Can you work these out from the drawing? Everything is in mm from the part's minimum corner. A direction names the side the tool comes from. Give positions to 0.01 mm unless a question says otherwise; leave off trailing zeros. Order: outer loops, then holes, each group sorted by start corner. A loop starts at its lowest first (then second) coordinate and runs counter-clockwise, first axis right, second up. Notation, with made-up numbers: M 82.25,-29 L 104.25,-29 A32 cw 104.25,10 Z; hole C -8,-25 d3. An arc over 180 degrees is marked long. Use a Markdown table: item, result. Add a question column.
Item 1: I'm going to push flat-ended pins straight in: pin 1 Ø5 at (x, z) = (42.5, 6) entering from +Y; pin 2 Ø16 at (x, y) = (37.5, 35) entering from +Z; pin 3 Ø2 at (x, z) = (22.5, 18) entering from +Y; pin 4 Ø10 at (x, y) = (35.5, 45) entering from -Z. Where does each tip first touch, or does it pass through?
Item 2: Suppose I cut it at C-C on y = 42.5. Write out the boundary of the cut face in (x, z).
Item 3: If I drill on L1, parallel to Y at x = 12.5, z = 44.5; L2, parallel to Z at x = 10, y = 7.5; L3, parallel to Z at x = 46.5, y = 44, over which ranges is the centre line in solid material (lowest first)? Write a range as from..to.
Item 4: Suppose I cut it at D-D on z = 12. Write out the boundary of the cut face in (x, y).
Item 5: If we mould it in two halves opening along X, with no side actions, what happens to the marked faces 1, 2 and 3? For each: released by +X, released by -X, zero draft, split by the parting line, or undercut.
Item 6: Suppose I cut it at B-B on z = 19. Write out the boundary of the cut face in (x, y), plus the area to 3 significant figures.
Item 7: For the marked faces 4, 5, 6 and 7, which set-ups out of +Z, -Z, +X, -X, +Y, -Y let a thin tool reach every point of the face, with its end or its side?
Item 8: Suppose I cut it at A-A on y = 13. Write out the boundary of the cut face in (x, z), plus the area to 3 significant figures.
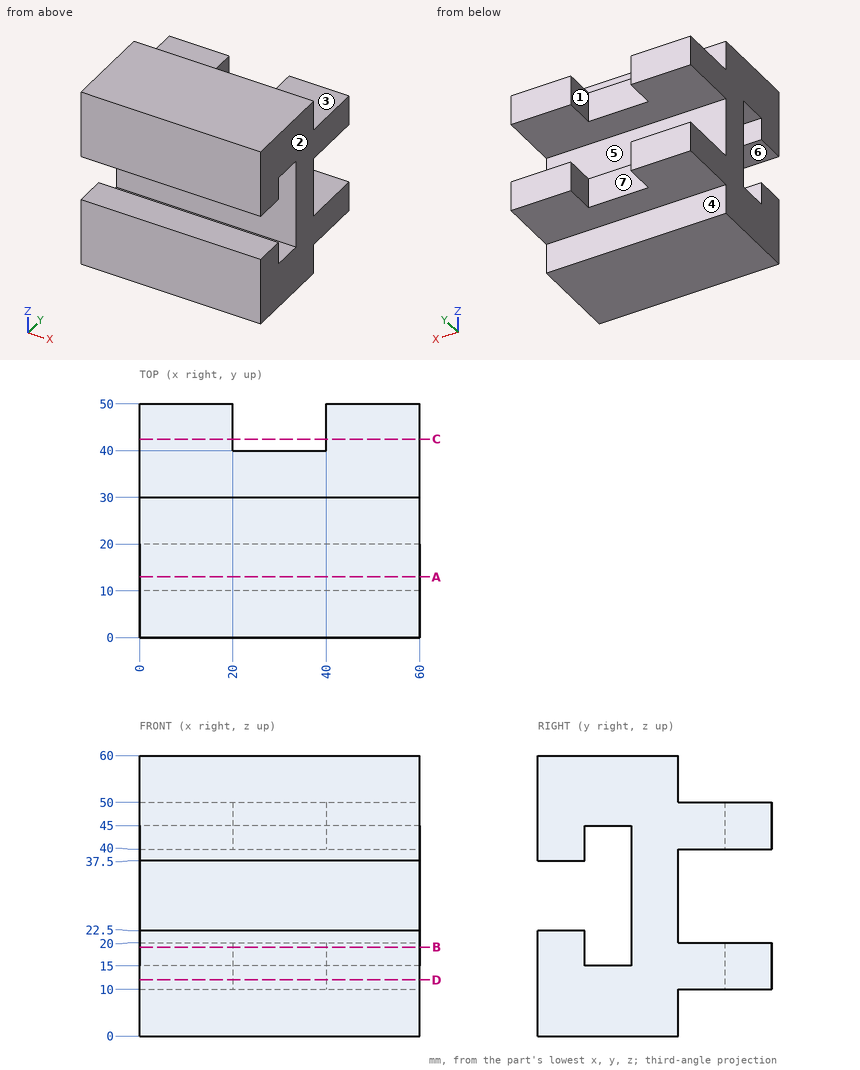
Findings below:
| question | item | result |
|---|---|---|
| 1 | pin 1 | stops at y = 30 |
| 1 | pin 2 | stops at z = 60 |
| 1 | pin 3 | stops at y = 40 |
| 1 | pin 4 | stops at z = 10 |
| 2 | outline | M 0,10 L 20,10 L 20,20 L 0,20 Z; M 0,40 L 20,40 L 20,50 L 0,50 Z; M 40,10 L 60,10 L 60,20 L 40,20 Z; M 40,40 L 60,40 L 60,50 L 40,50 Z |
| 3 | L1 | y = 0..10, 20..50 |
| 3 | L2 | z = 0..22.5, 37.5..60 |
| 3 | L3 | z = 10..20, 40..50 |
| 4 | outline | M 0,0 L 60,0 L 60,50 L 40,50 L 40,40 L 20,40 L 20,50 L 0,50 Z |
| 5 | face 1 | undercut |
| 5 | face 2 | released by +X |
| 5 | face 3 | zero draft |
| 6 | outline | M 0,0 L 60,0 L 60,10 L 0,10 Z; M 0,20 L 60,20 L 60,50 L 40,50 L 40,40 L 20,40 L 20,50 L 0,50 Z |
| 6 | area | 2,200 mm^2 |
| 7 | face 4 | -Z, +X, -X, +Y |
| 7 | face 5 | +X, -X, +Y |
| 7 | face 6 | +X, -X, -Y |
| 7 | face 7 | +Z, -Z, +Y |
| 8 | outline | M 0,0 L 60,0 L 60,15 L 0,15 Z; M 0,45 L 60,45 L 60,60 L 0,60 Z |
| 8 | area | 1,800 mm^2 |
